from build123d import *

# Parameters (mm, degrees)
BOSS_EXTRUDE1_DEPTH = 7.62
SKETCH2_R           = 8.5
BOSS_EXTRUDE2_DEPTH = 2
BOSS_EXTRUDE3_DEPTH = 2
CHAMFER1_SIZE       = 2
CHAMFER2_SIZE       = 1


with BuildPart() as part:
    # Sketch1 → Boss-Extrude1 (new body)
    with BuildSketch(Plane(origin=(0, 0, 0), x_dir=(1, 0, 0), z_dir=(0, 1, 0))):
        Polygon((3.723909236, 6.45), (-3.723909236, 6.45), (-7.447818473, 0), (-3.723909236, -6.45), (3.723909236, -6.45), (7.447818473, 0), align=None)
        with BuildLine():
            Line((-1.037493712, 1.218033989), (1.037493712, 1.218033989))
            ThreePointArc((1.037493712, 1.218033989), (0, -1.6), (-1.037493712, 1.218033989))
        make_face(mode=Mode.SUBTRACT)
    extrude(amount=BOSS_EXTRUDE1_DEPTH)

    # Sketch2 → Boss-Extrude2 (add)
    with BuildSketch(Plane.XZ):
        Circle(SKETCH2_R)
        with BuildLine():
            Line((1.037493712, -1.218033989), (-1.037493712, -1.218033989))
            ThreePointArc((-1.037493712, -1.218033989), (0, 1.6), (1.037493712, -1.218033989))
        make_face(mode=Mode.SUBTRACT)
    extrude(amount=BOSS_EXTRUDE2_DEPTH)

    # Sketch3 → Boss-Extrude3 (add)
    with BuildSketch(Plane(origin=(0, 7.62, 0), x_dir=(1, 0, 0), z_dir=(0, 1, 0))):
        Polygon((7.447818473, 0), (3.723909236, 6.45), (-3.723909236, 6.45), (-7.447818473, 0), (-3.723909236, -6.45), (3.723909236, -6.45), align=None)
        with BuildLine():
            Line((1.037493712, 1.218033989), (-1.037493712, 1.218033989))
            ThreePointArc((-1.037493712, 1.218033989), (0, -1.6), (1.037493712, 1.218033989))
        make_face(mode=Mode.SUBTRACT)
    extrude(amount=BOSS_EXTRUDE3_DEPTH)

    # Chamfer1
    chamfer1_edges = [part.edges().sort_by_distance(p)[0] for p in [
        (5.585863854, 9.62, 3.225),
        (5.585863854, 9.62, -3.225),
        (0, 9.62, -6.45),
        (-5.585863854, 9.62, -3.225),
        (-5.585863854, 9.62, 3.225),
        (0, 9.62, 6.45),
    ]]
    chamfer(chamfer1_edges, length=CHAMFER1_SIZE)

    # Chamfer2
    chamfer2_edges = [part.edges().sort_by_distance(p)[0] for p in [
        (0, -2, 1.6),
        (0, -2, -1.218033989),
    ]]
    chamfer(chamfer2_edges, length=CHAMFER2_SIZE)


solid = part.part
The model under review builds one solid part; all positions refer to its coordinate system, in mm. A direction names the side the tool comes from. Coordinates: 2 decimals unless noted, no trailing zeros. Loops run counter-clockwise (first coordinate to the right, second up) from the corner with the lowest first, then second, coordinate; pieces in that order, holes last. Notation, with made-up numbers: (-29, 83.5) -> (-4, 83.5) arc R19 ccw to (-4, 111.5) -> close; hole circle Ø6 at (0, 53). An arc over 180 degrees is marked (long way). Use a Markdown table: item, result. Add a question column.
1. Clearance check with flat-ended pins moving along their axes: pin 1 Ø2.5 at (x, y) = (0, 3) entering from +Z; pin 2 Ø3 at (x, z) = (-5, 5.5) entering from +Y; pin 3 Ø4 at (y, z) = (4, -0.5) entering from +X. State where each tip first meets the part, or that it passes through.
2. Machinability: for faces 1 (the face through (-5.6, 3.8, 3.2)), 2 (the face through (5.56, 3.76, 3.27)), 3 (the face through (0, 4, -1.218)), which of the approach directions +Z, -Z, +X, -X, +Y, -Y give a long, thin tool a straight path to every point of the face, cutting with its end or side? Answer none if there is none.
3. Add section B-B on y = 2.25. Write out the cut boundary in (x, z), plus the area to 3 significant figures.
4. Add section C-C on x = 6.25. Write out the cut boundary in (y, z).
5. Add section A-A on x = 0. Write out the cut boundary in (y, z), plus the area to 3 significant figures.
6. Add section D-D on z = -4. Write out the cut boundary in (x, y).
7. To check wall thickness, follow line 1 (Y direction, x = 7, z = 2.5); line 2 (Z direction, x = 0, y = -0.45); line 3 (Z direction, x = -0.75, y = -0.75). State the ranges of each line that lie inside material, in increasing order.
8. Draft analysis for pull direction X (two halves, no side actions). For faces 4 (the face through (4.57, -0.986, 7.167)), 5 (the face through (0.02, -1.51, -1.73)), 6 (the face through (-4.734, 8.634, 2.673)), state which applies: pulls with the +X half, pulls with the -X half, needs draft (parallel to the pull), parting line crosses it, or undercut.
Returned:
| question | item | result |
|---|---|---|
| 1 | pin 1 | stops at z = 6.45 |
| 1 | pin 2 | stops at y = 8.49 |
| 1 | pin 3 | stops at x = 7.45 |
| 2 | face 1 | +Z, -X, +Y |
| 2 | face 2 | +Z, +X, +Y |
| 2 | face 3 | +Y, -Y |
| 3 | outline | (-7.45, 0) -> (-3.72, -6.45) -> (3.72, -6.45) -> (7.45, 0) -> (3.72, 6.45) -> (-3.72, 6.45) -> close; hole (-1.04, -1.22) -> (1.04, -1.22) arc R1.6 ccw (long way) to start |
| 3 | area | 137 mm² |
| 4 | outline | (-2, -5.76) -> (0, -5.76) -> (0, -2.07) -> (7.62, -2.07) -> (8.66, 0) -> (7.62, 2.07) -> (0, 2.07) -> (0, 5.76) -> (-2, 5.76) -> close |
| 5 | outline | (-2, -8.5) -> (0, -8.5) -> (0, -6.45) -> (7.62, -6.45) -> (9.62, -4.45) -> (9.62, -1.22) -> (-1, -1.22) -> (-2, -2.22) -> close; (-2, 2.6) -> (-1, 1.6) -> (9.62, 1.6) -> (9.62, 4.45) -> (7.62, 6.45) -> (0, 6.45) -> (0, 8.5) -> (-2, 8.5) -> close |
| 5 | area | 120 mm² |
| 6 | outline | (-7.5, -2) -> (7.5, -2) -> (7.5, 0) -> (5.14, 0) -> (5.14, 7.62) -> (2.83, 9.62) -> (-2.83, 9.62) -> (-5.14, 7.62) -> (-5.14, 0) -> (-7.5, 0) -> close |
| 7 | line 1 | y = -2 to 0 |
| 7 | line 2 | z = -8.5 to -1.22, 1.6 to 8.5 |
| 7 | line 3 | z = -8.47 to -1.22, 1.41 to 8.47 |
| 8 | face 4 | parting line crosses it |
| 8 | face 5 | undercut |
| 8 | face 6 | pulls with the -X half |
